Design review of the part built by this model. Coordinates are the model's own, in mm. A direction names the side the tool comes from. Coordinates: 2 decimals unless noted, no trailing zeros. Loops run counter-clockwise (first coordinate to the right, second up) from the corner with the lowest first, then second, coordinate; pieces in that order, holes last. Notation, with made-up numbers: (45.25, 3.25) - (96.25, 3.25) arc R19 cw to (96.25, 8.25) - close; hole circle Ø3 at (63.25, -4.5). An arc over 180 degrees is marked (long way). Use one line per item in the form item = value. Start each with the question number.
(1) Add section C-C (z = 7.5). State the section outline as (x, y) points.
(2) Clearance check with flat-ended pins moving along their axes: pin 1 Ø5 at (x, y) = (-0.5, 11) entering from +Z; pin 2 Ø6 at (x, z) = (7.5, 53.5) entering from +Y; pin 3 Ø12 at (y, z) = (10.5, 45) entering from -X; pin 4 Ø6 at (y, z) = (-3, 44) entering from +X. State where each tip first meets the part, or that it passes through.
(3) Tool access review of faces 4 (the face through (0, -10, 56)), 5 (the face through (0, 10, 56)), 6 (the face through (0, -9, 55)), 7 (the face through (11.18, -4.63, 14.89)): name each direction out of +Z, -Z, +X, -X, +Y, -Y from which nothing blocks a thin tool from reaching the whole face with its end or side.
(4) Add section A-A (y = 0). State the section outline as (x, z) points.
(5) Add section D-D (x = 3.5). State the section outline as (y, z) points, plus the area to 3 significant figures.
(6) Add section B-B (x = 0). State the section outline as (y, z) points.
(7) The part is to be moulded in two halves that separate along Y. For faces 1 (the face through (0, 11, 55)), 2 (the face through (0, 0, 0)), 3 (the face through (-10.097, 9.259, 42.032)), say which applies: pulls with the +Y half, pulls with the -Y half, needs draft (parallel to the pull), parting line crosses it, or undercut.
(8) For L1, parallel to Z at x = -8, y = -5; L2, parallel to Z at x = 10.75, y = -8.25; L3, parallel to X at y = -6.25, z = 5, list the stretches that pass through material, from the lowest coordinate up.
```python
from build123d import *

# Parameters (mm, degrees)
SKETCH1_R           = 12.1
BOSS_EXTRUDE1_DEPTH = 30.2
SKETCH2_R           = 13.7
BOSS_EXTRUDE2_DEPTH = 24
SKETCH4_R           = 1
BOSS_EXTRUDE3_DEPTH = 1.8
SKETCH5_R           = 2.25
BOSS_EXTRUDE4_DEPTH = 22.3
CUT_EXTRUDE1_DEPTH  = 12


with BuildPart() as part:
    # Sketch1 → Boss-Extrude1 (new body)
    with BuildSketch(Plane.XY):
        Circle(SKETCH1_R)
    extrude(amount=BOSS_EXTRUDE1_DEPTH)

    # Sketch2 → Boss-Extrude2 (add)
    with BuildSketch(Plane.XY.offset(30.2)):
        Circle(SKETCH2_R)
    extrude(amount=BOSS_EXTRUDE2_DEPTH)

    # Sketch4 → Boss-Extrude3 (add)
    with BuildSketch(Plane.XY.offset(54.2)):
        with Locations((0, 10)):
            Circle(SKETCH4_R)
        with Locations((0, -10)):
            Circle(SKETCH4_R)
    extrude(amount=BOSS_EXTRUDE3_DEPTH)

    # Sketch5 → Boss-Extrude4 (add)
    with BuildSketch(Plane.XY.offset(54.2)):
        Circle(SKETCH5_R)
    extrude(amount=BOSS_EXTRUDE4_DEPTH)

    # Sketch6 → Cut-Extrude1 (cut)
    with BuildSketch(Plane.XY.offset(76.5)):
        Polygon((-55.042727248, 1.25), (-1.870828693, 1.25), (1.870828693, 1.25), (55.042727248, 1.25), (55.042727248, 107.593797109), (-55.042727248, 107.593797109), align=None)
    extrude(amount=-CUT_EXTRUDE1_DEPTH, mode=Mode.SUBTRACT)


solid = part.part
```
Computed values:
q1.outline = circle Ø24.2 at (0, 0)
q2.pin_1 = 56
q2.pin_2 = 12.94
q2.pin_3 = -12.94
q2.pin_4 = 13.7
q3.face_4 = +Z, +X, -X, -Y
q3.face_5 = +Z, +X, -X, +Y
q3.face_6 = +Z
q3.face_7 = -Z
q4.outline = (-13.7, 30.2) - (-12.1, 30.2) - (-12.1, 0) - (12.1, 0) - (12.1, 30.2) - (13.7, 30.2) - (13.7, 54.2) - (2.25, 54.2) - (2.25, 76.5) - (-2.25, 76.5) - (-2.25, 54.2) - (-13.7, 54.2) - close
q5.outline = (-13.25, 30.2) - (-11.58, 30.2) - (-11.58, 0) - (11.58, 0) - (11.58, 30.2) - (13.25, 30.2) - (13.25, 54.2) - (-13.25, 54.2) - close
q5.area = 1,340 mm^2
q6.outline = (-13.7, 30.2) - (-12.1, 30.2) - (-12.1, 0) - (12.1, 0) - (12.1, 30.2) - (13.7, 30.2) - (13.7, 54.2) - (11, 54.2) - (11, 56) - (9, 56) - (9, 54.2) - (2.25, 54.2) - (2.25, 64.5) - (1.25, 64.5) - (1.25, 76.5) - (-2.25, 76.5) - (-2.25, 54.2) - (-9, 54.2) - (-9, 56) - (-11, 56) - (-11, 54.2) - (-13.7, 54.2) - close
q7.face_1 = undercut
q7.face_2 = needs draft
q7.face_3 = parting line crosses it
q8.L1 = 0 to 54.2
q8.L2 = 30.2 to 54.2
q8.L3 = -10.36 to 10.36
